Model file for the job. Use its own axes, mm. Face numbers are marked on the shaded views. A direction names the side the tool comes from. Coordinates: 2 decimals unless noted, no trailing zeros. Order: outer loops, then holes, each group sorted by start corner. A loop starts at its lowest first (then second) coordinate and runs counter-clockwise, first axis right, second up.
Autodesk Fusion 360 part; units mm, degrees
sketch "main-upper" plane through (0, 0, 0) normal (0, 0, 1) x (1, 0, 0)
  line L0 (33.55, 18.7) -> (-33.55, 18.7)
  line L1 (-33.55, 18.7) -> (-33.55, -18.7)
  line L2 (-33.55, -18.7) -> (33.55, -18.7)
  line L3 (33.55, -18.7) -> (33.55, 18.7)
  line L4 (33.55, 18.7) -> (-33.55, -18.7) construction
  line L5 (-33.55, 18.7) -> (33.55, -18.7) construction
  dimension "d1" = 67.1
  dimension "d2" = 37.4
extrude "Extrude1" add sketch "main-upper" against normal blind 8 draft -3
sketch "rgb-led" plane through (0, 0, 0) normal (0, 0, 1) x (-1, 0, 0)
  line L0 (-33.55, 18.7) -> (-33.55, -18.7)
  line L1 (-33.55, -18.7) -> (33.55, -18.7)
  line L2 (33.55, -18.7) -> (33.55, 18.7)
  line L3 (33.55, 18.7) -> (-33.55, 18.7)
  line L4 (-27.8, -1) -> (-27.8, 1)
  arc A0 (-27.8, 1) -> (-29.05, 1) centre (-28.425, 1) ccw
  line L5 (-29.05, 1) -> (-29.05, -1)
  arc A1 (-29.05, -1) -> (-27.8, -1) centre (-28.425, -1) ccw
  line L6 (-28.425, -1.625) -> (-28.425, 1.625) construction
  line L7 (-28.425, -18.7) -> (-28.425, 18.7) construction
  point P0 (-28.425, 0)
  point P1 (-28.425, 0)
  dimension "d5" = 3.25
  dimension "d6" = 1.25
  dimension "d8" = 4.5
extrude "Extrude2" add sketch "rgb-led" along normal blind 0.6 contours L4 A0 L5 A1
fillet "Fillet1" radius 0.25 4 edges at (28.425, 1.625, 0.6) (27.8, 0, 0.6) (28.425, -1.625, 0.6) (29.05, 0, 0.6)
sketch "eink" plane through (0, 0, 0) normal (0, 0, 1) x (-1, 0, 0)
  line L0 (-29.05, -1) -> (-29.05, 1)
  arc A0 (-27.8, 1) -> (-29.05, 1) centre (-28.425, 1) ccw
  line L1 (-27.8, 1) -> (-27.8, -1)
  arc A1 (-29.05, -1) -> (-27.8, -1) centre (-28.425, -1) ccw
  line L2 (-33.55, 18.7) -> (-33.55, -18.7)
  line L3 (-33.55, -18.7) -> (33.55, -18.7)
  line L4 (33.55, -18.7) -> (33.55, 18.7)
  line L5 (33.55, 18.7) -> (-33.55, 18.7)
  line L6 (-24.05, 14) -> (24.05, 14)
  line L7 (24.05, 14) -> (24.05, -14)
  line L8 (24.05, -14) -> (-24.05, -14)
  line L9 (-24.05, -14) -> (-24.05, 14)
  line L10 (-24.05, 14) -> (24.05, -14) construction
  line L11 (24.05, 14) -> (-24.05, -14) construction
  dimension "d13" = 48.1
  dimension "d14" = 28
sketch "buttons-base" plane through (0, -18.6488, -0.9773) normal (0, -0.9986, -0.0523) x (1, 0, 0)
  line L0 (-33.1307, -7.0323) -> (33.1307, -7.0323)
  line L1 (33.1307, -7.0323) -> (33.55, 0.9787)
  line L2 (33.55, 0.9787) -> (-33.55, 0.9787)
  line L3 (-33.55, 0.9787) -> (-33.1307, -7.0323)
  line L4 (-27.65, -5.4713) -> (-4.95, -5.4713)
  arc A0 (-4.95, -5.4713) -> (-4.95, -0.6713) centre (-4.95, -3.0713) ccw
  line L5 (-4.95, -0.6713) -> (-27.65, -0.6713)
  arc A1 (-27.65, -0.6713) -> (-27.65, -5.4713) centre (-27.65, -3.0713) ccw
  line L6 (-30.05, -3.0713) -> (-2.55, -3.0713) construction
  dimension "d15" = 4.8
  dimension "d16" = 27.5
  dimension "d17" = 1.65
  dimension "d19" = 3.5
sketch "buttons" plane through (0, -18.6488, -0.9773) normal (0, -0.9986, -0.0523) x (1, 0, 0)
  line L0 (-27.15, -4.4713) -> (-21.95, -4.4713)
  arc A0 (-21.95, -4.4713) -> (-21.95, -1.6713) centre (-21.95, -3.0713) ccw
  line L1 (-21.95, -1.6713) -> (-27.15, -1.6713)
  arc A1 (-27.15, -1.6713) -> (-27.15, -4.4713) centre (-27.15, -3.0713) ccw
  line L2 (-28.55, -3.0713) -> (-20.55, -3.0713) construction
  line L3 (-30.05, -3.0713) -> (-2.55, -3.0713)
  line L4 (-27.65, -5.4713) -> (-4.95, -5.4713)
  line L5 (-16.3, -3.0713) -> (-16.3, -5.4713) construction
  line L6 (-5.45, -4.4713) -> (-10.65, -4.4713)
  arc A2 (-10.65, -1.6713) -> (-10.65, -4.4713) centre (-10.65, -3.0713) ccw
  line L7 (-10.65, -1.6713) -> (-5.45, -1.6713)
  arc A3 (-5.45, -4.4713) -> (-5.45, -1.6713) centre (-5.45, -3.0713) ccw
  dimension "d20" = 8
  dimension "d21" = 2.8
  dimension "d22" = 1.5
extrude "Extrude3" add sketch "buttons-base" along normal blind 0.1 contours L4 A0 L5 A1
extrude "Extrude4" add sketch "buttons" along normal blind 1.2
sketch "batery-compartment-body" plane through (0, 0, -8) normal (0, 0, -1) x (1, 0, 0)
  line L0 (-33.1307, -18.2807) -> (33.1307, -18.2807)
  line L1 (33.1307, -18.2807) -> (33.1307, 18.2807)
  line L2 (33.1307, 18.2807) -> (-33.1307, 18.2807)
  line L3 (-33.1307, 18.2807) -> (-33.1307, -18.2807)
  line L4 (-28.75, -15.7) -> (28.75, -15.7)
  line L5 (28.75, -15.7) -> (28.75, 15.7)
  line L6 (28.75, 15.7) -> (-28.75, 15.7)
  line L7 (-28.75, 15.7) -> (-28.75, -15.7)
  line L8 (-28.75, -15.7) -> (28.75, 15.7) construction
  line L9 (28.75, -15.7) -> (-28.75, 15.7) construction
  dimension "d27" = 57.5
  dimension "d28" = 31.4
extrude "Extrude5" add sketch "batery-compartment-body" along normal blind 5.4 draft -3 contours L4 L5 L6 L7
sketch "rear-label-indent" plane through (0, 0, -13.4) normal (0, 0, -1) x (1, 0, 0)
  line L0 (28.467, 15.417) -> (-28.467, 15.417)
  line L1 (-28.467, 15.417) -> (-28.467, -15.417)
  line L2 (-28.467, -15.417) -> (28.467, -15.417)
  line L3 (28.467, -15.417) -> (28.467, 15.417)
  line L4 (15.5, 12.5) -> (-15.5, 12.5)
  line L5 (-17.5, 10.5) -> (-17.5, -10.5)
  line L6 (-15.5, -12.5) -> (15.5, -12.5)
  line L7 (17.5, -10.5) -> (17.5, 10.5)
  line L8 (17.5, 12.5) -> (-17.5, -12.5) construction
  line L9 (-17.5, 12.5) -> (17.5, -12.5) construction
  line L10 (17.5, -10.5) -> (15.5, -12.5)
  line L11 (17.5, -12.5) -> (17.5, -10.5) construction
  line L12 (15.5, -12.5) -> (17.5, -12.5) construction
  arc A0 (-17.5, -10.5) -> (-15.5, -12.5) centre (-15.5, -10.5) ccw
  arc A1 (-15.5, 12.5) -> (-17.5, 10.5) centre (-15.5, 10.5) ccw
  arc A2 (17.5, 10.5) -> (15.5, 12.5) centre (15.5, 10.5) ccw
  dimension "d34" = 35
  dimension "d35" = 25
  dimension "d36" = 45
  dimension "d37" = 33
  dimension "d38" = 2
  dimension "d39" = 2
  dimension "d40" = 2
extrude "Extrude6" cut sketch "rear-label-indent" against normal blind 0.1 contours L4 L5 L6 L7 L10 A0 A1 A2
ref_plane "WorkPlane1" through (-28.467, 0, 0) normal (1, 0, 0) x (0, 1, 0)
sketch "clips-profiile" plane through (-28.467, 0, 0) normal (1, 0, 0) x (0, 1, 0)
  line L0 (15.417, -13.4) -> (-15.417, -13.4)
  line L1 (-15.417, -13.4) -> (-15.7, -8)
  line L2 (-15.7, -8) -> (15.7, -8)
  line L3 (15.7, -8) -> (15.417, -13.4)
  line L4 (-15.5218, -11.4) -> (-17.017, -11.4)
  line L5 (-17.017, -11.4) -> (-17.017, -12.4)
  line L6 (-17.017, -12.4) -> (-15.417, -13.4)
  line L7 (15.5218, -11.4) -> (17.267, -11.4)
  line L8 (17.267, -11.4) -> (17.267, -12.4)
  line L9 (17.267, -12.4) -> (15.417, -13.4)
  dimension "d49" = 2
  dimension "d50" = 1.6
  dimension "d51" = 1.85
  dimension "d52" = 1
  dimension "d53" = 1
fillet "Fillet2" radius 3 4 edges at (-33.3404, 18.4904, -4) (33.3404, 18.4904, -4) (33.3404, -18.4904, -4) (-33.3404, -18.4904, -4)
fillet "Fillet3" radius 3 4 edges at (28.6085, 15.5585, -10.7) (28.6085, -15.5585, -10.7) (-28.6085, -15.5585, -10.7) (-28.6085, 15.5585, -10.7)
extrude "Extrude7" add sketch "clips-profiile" along normal blind 48 from surface at 5 contours L3 L7 L8 L9 | L1 L4 L5 L6
sketch "clips-cut" plane through (0, 0, -11.4) normal (0, 0, 1) x (-1, 0, 0)
  line L0 (23.467, -17.267) -> (23.467, -15.5218)
  line L1 (23.467, -15.5218) -> (-24.533, -15.5218)
  line L2 (-24.533, -15.5218) -> (-24.533, -17.267)
  line L3 (-24.533, -17.267) -> (23.467, -17.267)
  line L4 (23.467, 15.5218) -> (23.467, 17.017)
  line L5 (23.467, 17.017) -> (-24.533, 17.017)
  line L6 (-24.533, 17.017) -> (-24.533, 15.5218)
  line L7 (-24.533, 15.5218) -> (23.467, 15.5218)
  line L8 (21.95, 18.6612) -> (27.15, 18.6612)
  line L9 (27.15, 18.6612) -> (27.15, 19.7597)
  line L10 (27.15, 19.7597) -> (21.95, 19.7597)
  line L11 (21.95, 19.7597) -> (21.95, 18.6612)
  line L12 (5.45, 18.6612) -> (10.65, 18.6612)
  line L13 (10.65, 18.6612) -> (10.65, 19.7597)
  line L14 (10.65, 19.7597) -> (5.45, 19.7597)
  line L15 (5.45, 19.7597) -> (5.45, 18.6612)
  line L16 (0, 0) -> (0, 30) construction
  line L17 (5, 15.5218) -> (5, 17.017)
  line L18 (15, 15.5218) -> (15, 17.017)
  line L19 (-15, 15.5218) -> (-15, 17.017)
  line L20 (-5, 15.5218) -> (-5, 17.017)
  line L21 (-10, -17.267) -> (-10, -15.5218)
  line L22 (10, -17.267) -> (10, -15.5218)
  line L23 (-1.25, -17.267) -> (-1.25, -15.5218)
  line L24 (1.25, -17.267) -> (1.25, -15.5218)
  dimension "d61" = 10
  dimension "d62" = 5
  dimension "d63" = 10
  dimension "d64" = 1.25
extrude "Extrude9" cut sketch "clips-cut" against normal blind 2 draft 3 contours L4 L5 L7 L18 | L5 L7 L17 L20 | L5 L6 L7 L19
extrude "Extrude10" cut sketch "clips-cut" against normal blind 2 draft 3 contours L0 L1 L3 L22 | L1 L3 L23 L24 | L1 L2 L3 L21
chamfer "Chamfer1" distance 1.5 angle 45 2 edges at (1.2762, 17.267, -11.9) (-1.2762, 17.267, -11.9)
sketch "battery-door-tabs" plane through (0, 0, -13.4) normal (0, 0, -1) x (1, 0, 0)
  arc A0 (17.5, 10.5) -> (15.5, 12.5) centre (15.5, 10.5) ccw
  line L0 (17.5, 10.5) -> (17.5, -10.5)
  line L1 (17.5, -10.5) -> (15.5, -12.5)
  line L2 (15.5, -12.5) -> (-15.5, -12.5)
  arc A1 (-17.5, -10.5) -> (-15.5, -12.5) centre (-15.5, -10.5) ccw
  line L3 (-17.5, -10.5) -> (-17.5, 10.5)
  arc A2 (-15.5, 12.5) -> (-17.5, 10.5) centre (-15.5, 10.5) ccw
  line L4 (-15.5, 12.5) -> (15.5, 12.5)
  ellipse E0 centre (-25.4629, -12.4129) end of major axis (-27.59, -14.54) minor radius 3 (-28.467, -12.4211) -> (-25.4711, -15.417) ccw
  line L5 (-25.4711, -15.417) -> (-9.8952, -15.417)
  line L6 (-9.8952, -15.417) -> (-1.3548, -15.417)
  line L7 (-1.3548, -15.417) -> (1.3548, -15.417)
  line L8 (1.3548, -15.417) -> (9.8952, -15.417)
  line L9 (9.8952, -15.417) -> (25.4711, -15.417)
  ellipse E1 centre (25.4629, -12.4129) end of major axis (27.59, -14.54) minor radius 3 (25.4711, -15.417) -> (28.467, -12.4211) ccw
  line L10 (28.467, -12.4211) -> (28.467, 12.4211)
  ellipse E2 centre (25.4629, 12.4129) end of major axis (27.59, 14.54) minor radius 3 (28.467, 12.4211) -> (25.4711, 15.417) ccw
  line L11 (25.4711, 15.417) -> (14.8952, 15.417)
  line L12 (14.8952, 15.417) -> (5.1048, 15.417)
  line L13 (5.1048, 15.417) -> (-5.1048, 15.417)
  line L14 (-5.1048, 15.417) -> (-14.8952, 15.417)
  line L15 (-14.8952, 15.417) -> (-25.4711, 15.417)
  ellipse E3 centre (-25.4629, 12.4129) end of major axis (-27.59, 14.54) minor radius 3 (-25.4711, 15.417) -> (-28.467, 12.4211) ccw
  line L16 (-28.467, 12.4211) -> (-28.467, -12.4211)
  line L17 (-5.1048, 15.417) -> (-5.0524, 17.017)
  line L18 (-5.0524, 17.017) -> (-14.9476, 17.017)
  line L19 (-14.9476, 17.017) -> (-14.8952, 15.417)
  line L20 (-14.8952, 15.417) -> (-5.1048, 15.417)
  line L21 (-15.8952, 15.417) -> (-21.8952, 15.417)
  line L22 (-21.8952, 15.417) -> (-21.8952, 16.217)
  line L23 (-21.8952, 16.217) -> (-15.8952, 16.217)
  line L24 (-15.8952, 16.217) -> (-15.8952, 15.417)
  line L25 (-15.8952, 15.417) -> (-21.8952, 16.217) construction
  line L26 (-21.8952, 15.417) -> (-15.8952, 16.217) construction
  line L27 (0, 0) -> (0, 15.417) construction
  line L28 (15.8952, 16.217) -> (15.8952, 15.417)
  line L29 (21.8952, 15.417) -> (21.8952, 16.217)
  line L30 (21.8952, 16.217) -> (15.8952, 16.217)
  point P0 (-18.8952, 15.817)
  dimension "d75" = 0.8
  dimension "d76" = 6
  dimension "d77" = 1
extrude "Extrude11" add sketch "battery-door-tabs" against normal blind 1.5 contours L15 L21 L22 L23 L24 | L11 L28 L29 L30
equation "d64 = ( 2.5 / 2 ) * 1 mm"
equation "d66 = body_draft_angle"
equation "d68 = body_draft_angle"
equation "d71 = corner_radius"
equation "d73 = corner_radius"
equation "corner_radius = 3.0 mm"
equation "body_draft_angle = 3 deg"
equation "pogo_pad = 1.5 mm"
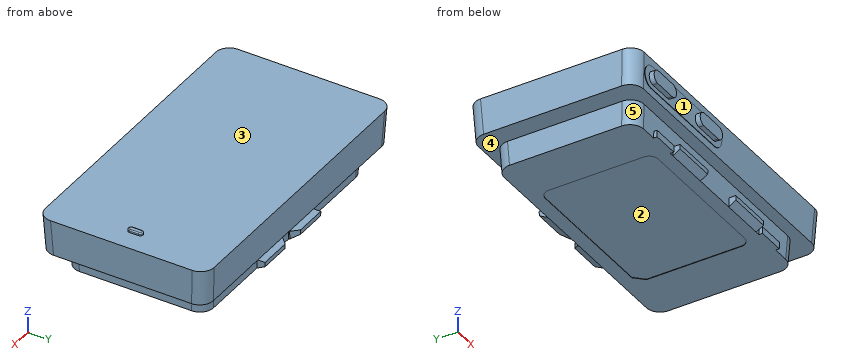
Q1. Which spindle directions (+Z, -Z, +X, -X, +Y, -Y) get a long thin tool onto all of the face, cutting with end or side? Do the marked faces 4 and 5. Say none if no direction does.
Established:
face 4: none
face 5: -Z, -X, -Y
Q2. Cut at B-B, the plane y = -9. List the corners of the cut face in (x, z), plus the area to 3 significant figures.
Established:
outline: (-33.55, 0) - (-33.13, -8) - (-28.75, -8) - (-28.47, -13.4) - (-17.5, -13.4) - (-17.5, -13.3) - (17.5, -13.3) - (17.5, -13.4) - (28.47, -13.4) - (28.75, -8) - (33.13, -8) - (33.55, 0) - close
area: 839 mm2
Q3. Cut at A-A, the plane x = 23. List the corners of the cut face in (y, z), plus the area to 3 significant figures.
Established:
outline: (-18.7, 0) - (-18.28, -8) - (-15.7, -8) - (-15.42, -13.4) - (15.42, -13.4) - (15.7, -8) - (18.28, -8) - (18.7, 0) - close
area: 464 mm2
Q4. Mould opens along Z. For the marked faces 1, 2 and 3 say: pulls with the +Z half, pulls with the -Z half, needs draft (parallel to the pull), parting line crosses it, or undercut.
Established:
face 1: undercut
face 2: pulls with the -Z half
face 3: pulls with the +Z half
Q5. Cut at C-C, the plane x = 12. List the corners of the cut face in (y, z).
Established:
outline: (-18.7, 0) - (-18.28, -8) - (-15.7, -8) - (-15.52, -11.4) - (-17.02, -11.4) - (-17.02, -12.4) - (-15.42, -13.4) - (-12.5, -13.4) - (-12.5, -13.3) - (12.5, -13.3) - (12.5, -13.4) - (15.42, -13.4) - (15.7, -8) - (18.28, -8) - (18.7, 0) - close
Q6. Cut at D-D, the plane x = -24.5. List the corners of the cut face in (y, z).
Established:
outline: (-19.76, -2.71) - (-19.61, -5.51) - (-18.51, -5.45) - (-18.46, -6.45) - (-18.36, -6.44) - (-18.28, -8) - (-15.7, -8) - (-15.42, -13.4) - (15.42, -13.4) - (15.7, -8) - (18.28, -8) - (18.7, 0) - (-18.7, 0) - (-18.61, -1.65) - (-18.71, -1.65) - (-18.66, -2.65) - close
Q7. Probe line 1 (Z direction, x = 25, y = 4); line 2 (X direction, y = -6.5, z = -0.25); line 3 (Y direction, x = -24.5, z = -11.5). List the from-to ranges inside material, lowest first.
Established:
line 1: z = -13.4 to 0
line 2: x = -33.54 to 33.54
line 3: y = -15.52 to 15.52
Q8. Drop flat-ended pins along their axis: P1, Ø1.1, axis at x = 11.5, z = -12, coming from the -Y side; P2, Ø5, axis at x = 1.5, z = -4, coming from the +Y side; P3, Ø1.4, axis at x = 7.5, y = 16, coming from the +Z side. Give the stop position or say it passes through.
Established:
P1: stops at y = -17.02
P2: stops at y = 18.62
P3: stops at z = 0
